from build123d import *

# Parameters (mm, degrees)
SKETCH_W        = 57
SKETCH_H        = 95
SKETCH_R        = 3.5
SKETCH_R_2      = 1.3
SKETCH_W_2      = 14.1
SKETCH_H_2      = 14.1
PAD_DEPTH       = 3
SKETCH008_R     = 2.5
POCKET_DEPTH    = 1
SKETCH009_W     = 3
SKETCH009_H     = 10
PAD002_DEPTH    = 6
SKETCH010_W     = 13
SKETCH010_H     = 15
POCKET006_DEPTH = 2
SKETCH011_W     = 10
SKETCH011_H     = 3
PAD003_DEPTH    = 10
FILLET_R        = 1


with BuildPart() as part:
    # Sketch → Pad (new body)
    with BuildSketch(Plane.XY):
        with Locations((28.5, 47.5)):
            Rectangle(SKETCH_W, SKETCH_H)
        with Locations((9.5, 47.5)):
            Circle(SKETCH_R, mode=Mode.SUBTRACT)
        with Locations((19, 85.5)):
            Circle(SKETCH_R_2, mode=Mode.SUBTRACT)
        with Locations((38, 85.5)):
            Circle(SKETCH_R_2, mode=Mode.SUBTRACT)
        with Locations((38, 66.5)):
            Circle(SKETCH_R_2, mode=Mode.SUBTRACT)
        with Locations((19, 66.5)):
            Circle(SKETCH_R_2, mode=Mode.SUBTRACT)
        with Locations((38, 28.5)):
            Circle(SKETCH_R_2, mode=Mode.SUBTRACT)
        with Locations((19, 28.5)):
            Circle(SKETCH_R_2, mode=Mode.SUBTRACT)
        with Locations((19, 9.5)):
            Circle(SKETCH_R_2, mode=Mode.SUBTRACT)
        with Locations((38, 9.5)):
            Circle(SKETCH_R_2, mode=Mode.SUBTRACT)
        with Locations((47.5, 19)):
            Circle(SKETCH_R_2, mode=Mode.SUBTRACT)
        with Locations((47.5, 76)):
            Circle(SKETCH_R_2, mode=Mode.SUBTRACT)
        with Locations((9.5, 9.5)):
            Rectangle(SKETCH_W_2, SKETCH_H_2, mode=Mode.SUBTRACT)
        with Locations((28.5, 9.5)):
            Rectangle(SKETCH_W_2, SKETCH_H_2, mode=Mode.SUBTRACT)
        with Locations((47.5, 9.5)):
            Rectangle(SKETCH_W_2, SKETCH_H_2, mode=Mode.SUBTRACT)
        with Locations((47.5, 28.5)):
            Rectangle(SKETCH_W_2, SKETCH_H_2, mode=Mode.SUBTRACT)
        with Locations((47.5, 66.5)):
            Rectangle(SKETCH_W_2, SKETCH_H_2, mode=Mode.SUBTRACT)
        with Locations((47.5, 85.5)):
            Rectangle(SKETCH_W_2, SKETCH_H_2, mode=Mode.SUBTRACT)
        with Locations((28.5, 85.5)):
            Rectangle(SKETCH_W_2, SKETCH_H_2, mode=Mode.SUBTRACT)
        with Locations((9.5, 85.5)):
            Rectangle(SKETCH_W_2, SKETCH_H_2, mode=Mode.SUBTRACT)
    extrude(amount=PAD_DEPTH)

    # Sketch008 (on Face49 of Pad) → Pocket (cut)
    with BuildSketch(Plane.XY.offset(3)):
        with Locations((19, 28.5)):
            Circle(SKETCH008_R)
        with Locations((38, 28.5)):
            Circle(SKETCH008_R)
        with Locations((47.5, 19)):
            Circle(SKETCH008_R)
        with Locations((38, 9.5)):
            Circle(SKETCH008_R)
        with Locations((19, 9.5)):
            Circle(SKETCH008_R)
        with Locations((19, 66.5)):
            Circle(SKETCH008_R)
        with Locations((38, 85.5)):
            Circle(SKETCH008_R)
        with Locations((38, 66.5)):
            Circle(SKETCH008_R)
        with Locations((47.5, 76)):
            Circle(SKETCH008_R)
        with Locations((19, 85.5)):
            Circle(SKETCH008_R)
    extrude(amount=-POCKET_DEPTH, mode=Mode.SUBTRACT)

    # Sketch009 (on Face4 of Pocket) → Pad002 (join)
    with BuildSketch(Plane(origin=(0, 0, 0), x_dir=(1, 0, 0), z_dir=(0, 0, -1))):
        with Locations((22.1, -47.5)):
            Rectangle(SKETCH009_W, SKETCH009_H)
    extrude(amount=PAD002_DEPTH)

    # Sketch010 (on Face4 of Pad002) → Pocket006 (cut)
    with BuildSketch(Plane(origin=(0, 0, 0), x_dir=(1, 0, 0), z_dir=(0, 0, -1))):
        with Locations((9.5, -47.5)):
            Rectangle(SKETCH010_W, SKETCH010_H)
    extrude(amount=-POCKET006_DEPTH, mode=Mode.SUBTRACT)

    # Sketch011 (on Face32 of Pocket006) → Pad003 (join)
    with BuildSketch(Plane.YZ.offset(23.6)):
        with Locations((47.5, -4.5)):
            Rectangle(SKETCH011_W, SKETCH011_H)
    extrude(amount=PAD003_DEPTH)

    # Fillet
    fillet_edges = [part.edges().sort_by_distance(p)[0] for p in [
        (57, 0, 1.5),
        (0, 0, 1.5),
        (0, 95, 1.5),
        (57, 95, 1.5),
    ]]
    fillet(fillet_edges, radius=FILLET_R)


with BuildPart() as part_1:
    # Body placement: moved
    add(part.part.moved(Location((6, 6, 11))))


solid = part_1.part
The model under review builds one solid part; all positions refer to its coordinate system, in mm. A direction names the side the tool comes from. Give positions to 0.01 mm unless a question says otherwise; leave off trailing zeros. Order: outer loops, then holes, each group sorted by start corner. A loop starts at its lowest first (then second) coordinate and runs counter-clockwise, first axis right, second up. Notation, with made-up numbers: (22.5, 82.5) -> (53.5, 82.5) arc R8 ccw to (53.5, 91.5) -> close; hole circle Ø11 at (-16, 11). An arc over 180 degrees is marked (long way). Write item = value, one per line. Start each with the question number.
(1) For pin 1 Ø4 at (x, y) = (44, 91.5) entering from +Z; pin 2 Ø0.9 at (y, z) = (51, 6.5) entering from +X; pin 3 Ø4 at (x, y) = (52, 77.5) entering from -Z, all flat-tipped, find the tip position at first contact; note any pin that passes through.
(2) Draft analysis for pull direction Y (two halves, no side actions). For faces 1 (the flat face through (6, 53, 12)), 2 (the flat face through (46.45, 91, 12)), state which applies: +Y half, -Y half, draft (parallel to the pull), parting line (faces both ways), or undercut.
(3) For L1, parallel to Y at x = 25, z = 11.7; L2, parallel to Y at x = 15.5, z = 13.25; L3, parallel to X at y = 72.5, z = 12, list the stretches that pass through material, from the lowest coordinate up. Write a range as from..to.
(4) Take a section at B-B (x = 32.5). Write out the cut boundary in (y, z).
(5) Take a section at D-D (x = 44). State how many separate pieces and enclosed holes the cut face has, plus the area to 3 significant figures.
(6) Tool access review of faces 3 (the flat face through (46.45, 72, 12)), 4 (the cylindrical face through (51, 25, 13.5)), 5 (the flat face through (22, 54, 12)): name each direction out of +Z, -Z, +X, -X, +Y, -Y from which nothing blocks a thin tool from reaching the whole face with its end or side.
(7) Take a section at C-C (y = 82). Write out the cut boundary in (x, z), plus the area to 3 significant figures.
(8) Take a section at A-A (y = 53.5). Write out the cut boundary in (x, z).
Returned:
q1.pin_1 = 13
q1.pin_2 = 39.6
q1.pin_3 = through
q2.face_1 = draft
q2.face_2 = undercut
q3.L1 = 6..14.2, 16.8..33.2, 35.8..71.2, 73.8..90.2, 92.8..101
q3.L2 = 6..8.45, 22.55..50, 57..84.45, 98.55..101
q3.L3 = 6..23.7, 26.3..42.7, 45.3..46.45, 60.55..63
q4.outline = (6, 11) -> (8.45, 11) -> (8.45, 14) -> (6, 14) -> close; (22.55, 11) -> (84.45, 11) -> (84.45, 14) -> (22.55, 14) -> close; (48.5, 5) -> (58.5, 5) -> (58.5, 8) -> (48.5, 8) -> close; (98.55, 11) -> (101, 11) -> (101, 14) -> (98.55, 14) -> close
q5.separate_pieces = 5
q5.enclosed_holes = 0
q5.area = 244 mm²
q6.face_3 = +Z, -Z
q6.face_4 = +Z
q6.face_5 = -Z
q7.outline = (6, 11) -> (52.2, 11) -> (52.2, 13) -> (51, 13) -> (51, 14) -> (6, 14) -> close; (54.8, 11) -> (63, 11) -> (63, 14) -> (56, 14) -> (56, 13) -> (54.8, 13) -> close
q7.area = 161 mm²
q8.outline = (6, 11) -> (9, 11) -> (9, 13) -> (12, 13) -> (12, 14) -> (6, 14) -> close; (19, 13) -> (22, 13) -> (22, 11) -> (26.6, 11) -> (26.6, 5) -> (39.6, 5) -> (39.6, 8) -> (29.6, 8) -> (29.6, 11) -> (63, 11) -> (63, 14) -> (19, 14) -> close
